Geometry: see drawing. Coordinates: mm, zero at the bounding-box minimum. A direction names the side the tool comes from. Round coordinates to 2 decimals unless told otherwise and drop trailing zeros. Order: outer loops, then holes, each group sorted by start corner. A loop starts at its lowest first (then second) coordinate and runs counter-clockwise, first axis right, second up. Notation, with made-up numbers: (-35, 16.5) -> (-15, 16.5) arc R17 ccw to (-15, 34.5) -> close; hole circle Ø4 at (64, -35.75). An arc over 180 degrees is marked (long way). One line per item, written item: value. Start each with the question number.
1) Pin query (flat end, axial travel): P1, Ø8, axis at x = 80, y = 34, coming from the +Z side; P2, Ø10, axis at y = 43.5, z = 38, coming from the -X side; P3, Ø10, axis at x = 118, y = 38, coming from the -Z side. Return the tip coordinate at first contact, or that it passes through.
2) Ray query, L1, parallel to Z at x = 75, y = 44.5; L2, parallel to Y at x = 56, z = 108; L3, parallel to X at y = 23, z = 66. Return the intervals inside material, ascending.
3) Section D-D (z = 53). Return the cut outline in (x, y), and give its area (3 significant figures).
4) Section B-B (x = 75). Return the cut outline in (y, z).
5) Reachability of the marked faces 1, 2 and 3 from +Z, -Z, +X, -X, +Y, -Y: full face, straight path, thin tool, end or side. Return the list, or none.
6) Section C-C (y = 39.5). Return the cut outline in (x, z).
7) Section A-A (z = 75). Return the cut outline in (x, y), and give its area (4 significant figures).
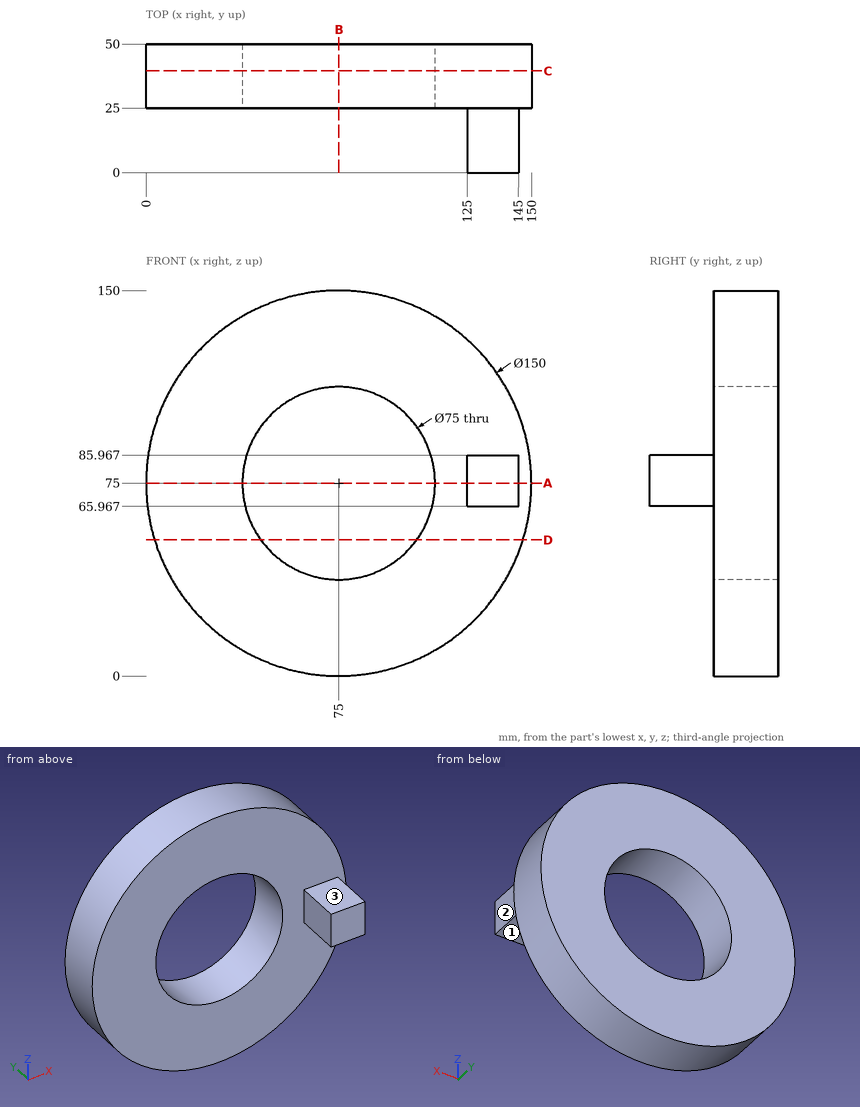
Findings:
1. P1: z = 149.99
1. P2: x = 7.17
1. P3: z = 10.34
2. L1: 0 to 37.5, 112.5 to 150
2. L2: 25 to 50
2. L3: 125 to 145
3. outline: (3.3, 25) -> (44.63, 25) -> (44.63, 50) -> (3.3, 50) -> close; (105.37, 25) -> (146.7, 25) -> (146.7, 50) -> (105.37, 50) -> close
3. area: 2,070 mm2
4. outline: (25, 0) -> (50, 0) -> (50, 37.5) -> (25, 37.5) -> close; (25, 112.5) -> (50, 112.5) -> (50, 150) -> (25, 150) -> close
5. face 1: -Z, +X, -X, -Y
5. face 2: +Z, -Z, +X, -Y
5. face 3: +Z, +X, -X, -Y
6. outline: circle Ø150 at (75, 75); hole circle Ø75 at (75, 75)
7. outline: (0, 25) -> (37.5, 25) -> (37.5, 50) -> (0, 50) -> close; (112.5, 25) -> (125, 25) -> (125, 0) -> (145, 0) -> (145, 25) -> (150, 25) -> (150, 50) -> (112.5, 50) -> close
7. area: 2,375 mm2
